```python
from build123d import *

# Parameters (mm, degrees)
SKETCH1_W           = 31.75
SKETCH1_H           = 165.1
BOSS_EXTRUDE1_DEPTH = 12.7
BOSS_EXTRUDE2_DEPTH = 12.7


with BuildPart() as part:
    # Sketch1 → Boss-Extrude1 (new body)
    with BuildSketch(Plane.XY):
        Rectangle(SKETCH1_W, SKETCH1_H)
    extrude(amount=BOSS_EXTRUDE1_DEPTH)

    # Sketch2 → Boss-Extrude2 (add)
    with BuildSketch(Plane.XY.offset(12.7)):
        with BuildLine():
            Line((15.875, 82.55), (28.575, 82.55))
            ThreePointArc((28.575, 82.55), (19.594743879, 78.830256121), (15.875, 69.85))
            Line((15.875, 69.85), (15.875, 82.55))
        make_face()
        with BuildLine():
            Line((15.875, -82.55), (15.875, -69.85))
            ThreePointArc((15.875, -69.85), (19.594743879, -78.830256121), (28.575, -82.55))
            Line((28.575, -82.55), (15.875, -82.55))
        make_face()
    extrude(amount=-BOSS_EXTRUDE2_DEPTH)


solid = part.part
```
Source: CAD feature listing. Evaluate the final solid. Frame: model axes, mm. A direction names the side the tool comes from. Round coordinates to 2 decimals unless told otherwise and drop trailing zeros. Write each loop counter-clockwise with the first axis right and the second up, starting at its lowest first coordinate (ties: lowest second). Pieces come first, ordered by that corner, then holes. Notation, with made-up numbers: M 37,87 L 70,87 A27 cw 70,122 Z; hole C -21.75,67.25 d10. An arc over 180 degrees is marked long. Use CSV: the item, a comma, the result in double quotes. Start each with the question number.
Q1. Cut plane C-C on y = -30. Output: boundary loops of the cut face in (x, z) (3 decimals).
Q2. Cut plane A-A on x = 22.5. Output: boundary loops of the cut face in (y, z).
Q3. Cut plane B-B on z = 7.5. Output: boundary loops of the cut face in (x, y) (3 decimals), plus the area to 3 significant figures.
Q4. Line query: line 1 (X direction, y = 9.5, z = 5) (3 decimals); line 2 (Y direction, x = 25.5, z = 4.5); line 3 (Y direction, x = 17, z = 2.75). Output: solid intervals per line, ascending. Write a range as from..to.
Q5. Pull-direction query (Y, two-part tool) for faces 3 (the face through (2, 1, 0)), 4 (the face through (6, -82.55, 6)), 5 (the face through (19.694, 78.928, 6.439)); classes: +Y half, -Y half, draft (parallel to the pull), parting line (faces both ways), or undercut.
Q6. Access query for faces 1 (the face through (-15.875, -1, 6)), 2 (the face through (19.497, -78.731, 6.439)). Directions: +Z, -Z, +X, -X, +Y, -Y. A direction counts if a zero-diameter tool reaches every point of the face in a straight line with its end or side. Return the directions, or none.
Q7. First-contact query: P1, Ø6, axis at y = 51, z = 5.5, coming from the +X side (3 decimals). Flat tip, straight axial feed; report the tip coordinate or a pass-through.
Results found:
1,outline,"M -15.875,0 L 15.875,0 L 15.875,12.7 L -15.875,12.7 Z"
2,outline,"M -82.55,0 L -81,0 L -81,12.7 L -82.55,12.7 Z; M 81,0 L 82.55,0 L 82.55,12.7 L 81,12.7 Z"
3,outline,"M -15.875,-82.55 L 28.575,-82.55 A12.7 cw 15.875,-69.85 L 15.875,69.85 A12.7 cw 28.575,82.55 L -15.875,82.55 Z"
3,area,"5,310 mm^2"
4,line 1,"-15.875..15.875"
4,line 2,"-82.55..-82.17, 82.17..82.55"
4,line 3,"-82.55..-75.08, 75.08..82.55"
5,face 3,"draft"
5,face 4,"-Y half"
5,face 5,"undercut"
6,face 1,"+Z, -Z, -X, +Y, -Y"
6,face 2,"+Z, -Z, +X"
7,P1,"x = 15.875"
